```python
from build123d import *

# Parameters (mm, degrees)
F0_R     = 2.5
F1_DEPTH = 2
F2_R     = 5


with BuildPart() as f1:
    # F0 (on Top) → F1 (new body)
    with BuildSketch(Plane.XY):
        Polygon((0, 150), (0, 0), (80, 0), (30, 150), align=None)
        with Locations((15, 135)):
            Circle(F0_R, mode=Mode.SUBTRACT)
    extrude(amount=F1_DEPTH)

    # F2
    f2_edges = [f1.edges().sort_by_distance(p)[0] for p in [
        (0, 150, 1),
        (30, 150, 1),
    ]]
    fillet(f2_edges, radius=F2_R)


solid = f1.part
```
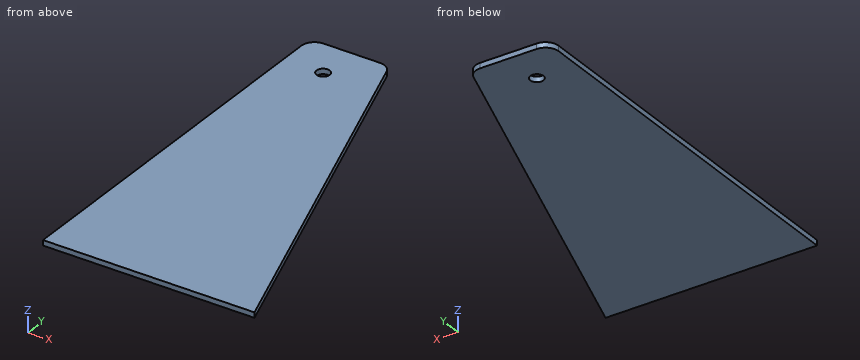
Verification items for the finished model (mm, model axes). Round coordinates to 2 decimals unless told otherwise and drop trailing zeros. Order: outer loops, then holes, each group sorted by start corner. A loop starts at its lowest first (then second) coordinate and runs counter-clockwise, first axis right, second up. Notation, with made-up numbers: (18, -3) - (26, -3) arc R22 cw to (26, 4) - close; hole circle Ø7 at (-33.75, 85.5). An arc over 180 degrees is marked (long way). Use CSV: the item, a comma, the result in double quotes. Start each with the question number.
1) Section check C-C, the plane y = 135. Record the cut outline in (x, z), plus the area to 3 significant figures.
2) Section check A-A, the plane x = 15. Record the cut outline in (y, z).
3) Section check D-D, the plane x = 38.5. Record the cut outline in (y, z), plus the area to 3 significant figures.
4) Thickness scan on L1, parallel to Y at x = 15, z = 0.8; L2, parallel to X at y = 135, z = 1; L3, parallel to X at y = 91.5, z = 0.5. Record the ranges inside material, lowest first.
5) Section check B-B, the plane z = 0.3. Record the cut outline in (x, y).
Answers:
1,outline,"(0, 0) - (12.5, 0) - (12.5, 2) - (0, 2) - close; (17.5, 0) - (35, 0) - (35, 2) - (17.5, 2) - close"
1,area,"60.0 mm²"
2,outline,"(0, 0) - (132.5, 0) - (132.5, 2) - (0, 2) - close; (137.5, 0) - (150, 0) - (150, 2) - (137.5, 2) - close"
3,outline,"(0, 0) - (124.5, 0) - (124.5, 2) - (0, 2) - close"
3,area,"249 mm²"
4,L1,"y = 0 to 132.5, 137.5 to 150"
4,L2,"x = 0 to 12.5, 17.5 to 35"
4,L3,"x = 0 to 49.5"
5,outline,"(0, 0) - (80, 0) - (31.14, 146.58) arc R5 ccw to (26.4, 150) - (5, 150) arc R5 ccw to (0, 145) - close; hole circle Ø5 at (15, 135)"
